Part print with two shaded views. Sizes in mm from the minimum x, y, z corner. A direction names the side the tool comes from. Round coordinates to 2 decimals unless told otherwise and drop trailing zeros. Loops run counter-clockwise (first coordinate to the right, second up) from the corner with the lowest first, then second, coordinate; pieces in that order, holes last. Notation, with made-up numbers: (-18, -37.75) -> (-11, -37.75) arc R11 cw to (-11, -16.75) -> close; hole circle Ø3 at (3, -35.75). An arc over 180 degrees is marked (long way). Use a Markdown table: item, result. Add a question column.
Item 1: Probe line 1 (Z direction, x = 37, y = 0.45); line 2 (X direction, y = 0.55, z = 27); line 3 (X direction, y = 2.25, z = 18). List the from-to ranges inside material, lowest first. Write a range as [from, to].
Item 2: Two-plate mould, pull along X, no slides. Class the marked faces 1, 2 and 3: pulls with the +X half, pulls with the -X half, needs draft (parallel to the pull), parting line crosses it, or undercut.
Item 3: Cut at A-A, the plane x = 3. List the corners of the cut face in (y, z).
Item 4: Flat gauge pins, fed straight in: pin 1 (1.6 mm diameter, centred on x = 3, z = 27, fed in from -Y); pin 2 (1.5 mm diameter, centred on x = 2, z = 15.5, fed in from +Y); pin 3 (1.2 mm diameter, centred on x = 2, y = 3.5, fed in from -Z); pin 4 (5.5 mm diameter, centred on x = 19.5, y = 5, fed in from -Z). Where does each tip first touch, or does it go through?
Item 5: Cut at C-C, the plane z = 18.25. List the corners of the cut face in (x, y), plus the area to 3 significant figures.
Item 6: Cut at D-D, the plane y = 9. List the corners of the cut face in (x, z), plus the area to 3 significant figures.
Item 7: Cut at B-B, the plane z = 27. List the corners of the cut face in (x, y).
Item 8: Which spindle directions (+Z, -Z, +X, -X, +Y, -Y) get a long thin tool onto all of the face, cutting with end or side? Do the marked faces 4, 5, 6 and 7. Say none if no direction does.
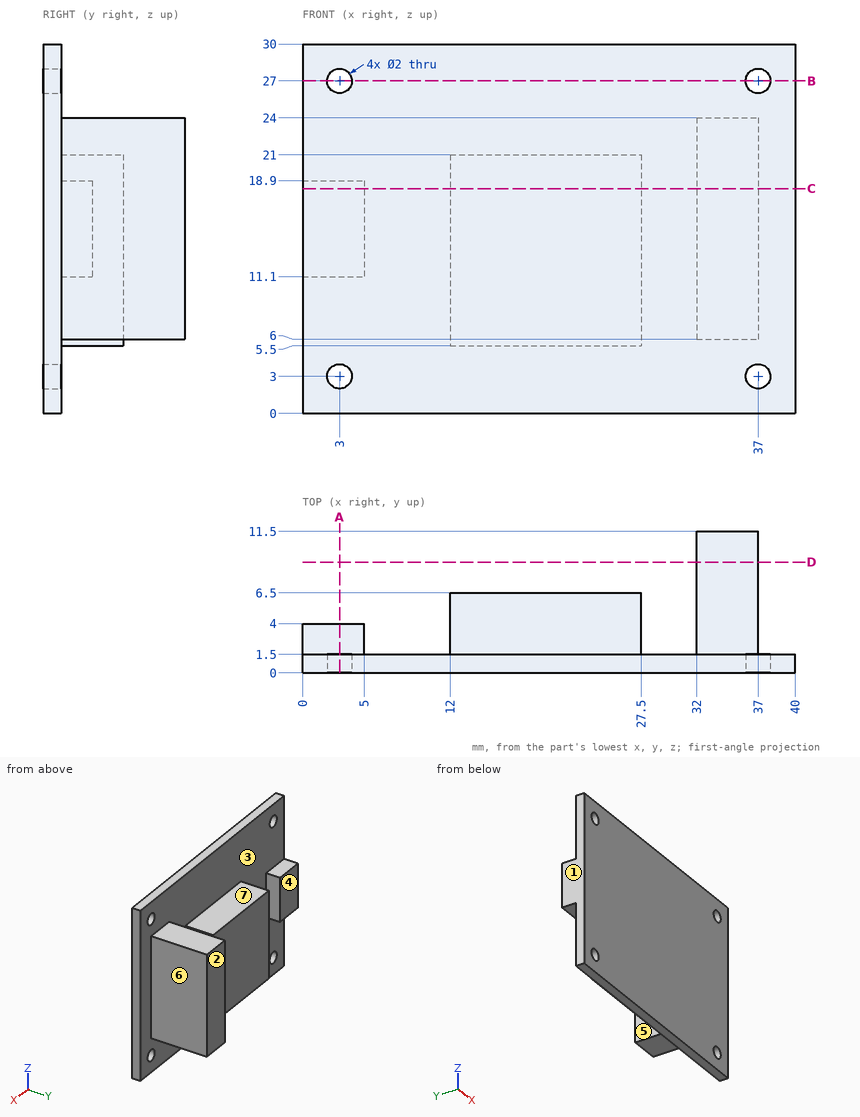
A:
| question | item | result |
|---|---|---|
| 1 | line 1 | z = [0, 2], [4, 26], [28, 30] |
| 1 | line 2 | x = [0, 2], [4, 36], [38, 40] |
| 1 | line 3 | x = [0, 5], [12, 27.5], [32, 37] |
| 2 | face 1 | pulls with the -X half |
| 2 | face 2 | needs draft |
| 2 | face 3 | undercut |
| 3 | outline | (0, 0) -> (1.5, 0) -> (1.5, 2) -> (0, 2) -> close; (0, 4) -> (1.5, 4) -> (1.5, 11.1) -> (4, 11.1) -> (4, 18.9) -> (1.5, 18.9) -> (1.5, 26) -> (0, 26) -> close; (0, 28) -> (1.5, 28) -> (1.5, 30) -> (0, 30) -> close |
| 4 | pin 1 | passes through |
| 4 | pin 2 | stops at y = 4 |
| 4 | pin 3 | stops at z = 11.1 |
| 4 | pin 4 | stops at z = 5.5 |
| 5 | outline | (0, 0) -> (40, 0) -> (40, 1.5) -> (37, 1.5) -> (37, 11.5) -> (32, 11.5) -> (32, 1.5) -> (27.5, 1.5) -> (27.5, 6.5) -> (12, 6.5) -> (12, 1.5) -> (5, 1.5) -> (5, 4) -> (0, 4) -> close |
| 5 | area | 200 mm^2 |
| 6 | outline | (32, 6) -> (37, 6) -> (37, 24) -> (32, 24) -> close |
| 6 | area | 90.0 mm^2 |
| 7 | outline | (0, 0) -> (2, 0) -> (2, 1.5) -> (0, 1.5) -> close; (4, 0) -> (36, 0) -> (36, 1.5) -> (4, 1.5) -> close; (38, 0) -> (40, 0) -> (40, 1.5) -> (38, 1.5) -> close |
| 8 | face 4 | +Z, -Z, -X, +Y |
| 8 | face 5 | +Z, -Z, +Y |
| 8 | face 6 | +Z, -Z, +X, +Y |
| 8 | face 7 | +Z, -X, +Y |
